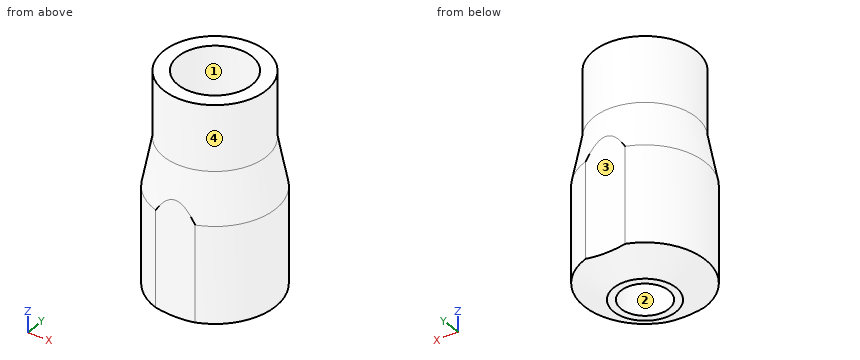
from build123d import *

# Parameters (mm, degrees)
SKETCH1_R           = 5.2451
BOSS_EXTRUDE1_DEPTH = 9.7155
CHAMFER1_SIZE       = 2.54
CHAMFER1_SIZE2      = 1.407944991
SKETCH2_R           = 4.445
SKETCH3_R           = 4.445
BOSS_EXTRUDE2_DEPTH = 5.6515
SKETCH4_R           = 2.069853247
CUT_EXTRUDE1_DEPTH  = 13.7795
SKETCH5_OUTSIDE_W   = 17.394
SKETCH5_OUTSIDE_H   = 17.394
SKETCH5_OUTSIDE_W_2 = 15.169695532
SKETCH5_OUTSIDE_H_2 = 9.924235678
CUT_EXTRUDE2_DEPTH  = 11.7475
SKETCH6_R           = 3.20242673
CUT_EXTRUDE3_DEPTH  = 8.1915


with BuildPart() as part:
    # Sketch1 → Boss-Extrude1 (new body)
    with BuildSketch(Plane.XY):
        with Locations(Location((0, 0, 0), (0, 0, 180))):
            Circle(SKETCH1_R)
    extrude(amount=BOSS_EXTRUDE1_DEPTH)

    # Chamfer1
    chamfer1_edges = [part.edges().sort_by_distance(p)[0] for p in [
        (5.2451, 0, 0),
    ]]
    chamfer1_side = [part.faces().sort_by_distance(p)[0] for p in [
        (0, 0, 0),
    ]]
    chamfer(chamfer1_edges, length=CHAMFER1_SIZE, length2=CHAMFER1_SIZE2, reference=chamfer1_side[0])

    # Sketch2 → section 1 of loft1
    with BuildSketch(Plane.XY.offset(13.8684), mode=Mode.PRIVATE) as loft1_s1:
        Circle(SKETCH2_R)
    # loft up to a face of the part (loft1)
    loft([Face(Wire([part.edges().sort_by_distance((3.590518025, -3.823513348, 9.7155))[0]])), loft1_s1.sketch])

    # Sketch3 → Boss-Extrude2 (add)
    with BuildSketch(Plane.XY.offset(13.8684)):
        with Locations(Location((0, 0, 0), (0, 0, 180))):
            Circle(SKETCH3_R)
    extrude(amount=BOSS_EXTRUDE2_DEPTH)

    # Sketch4 → Cut-Extrude1 (cut)
    with BuildSketch(Plane(origin=(0, 0, 0), x_dir=(-1, 0, 0), z_dir=(0, 0, -1))):
        Circle(SKETCH4_R)
    extrude(amount=-CUT_EXTRUDE1_DEPTH, mode=Mode.SUBTRACT)

    # Sketch5 outside → Cut-Extrude2 (cut)
    with BuildSketch(Plane.XY):
        Rectangle(SKETCH5_OUTSIDE_W, SKETCH5_OUTSIDE_H)
        with Locations((-0.203425036, 0)):
            Rectangle(SKETCH5_OUTSIDE_W_2, SKETCH5_OUTSIDE_H_2, mode=Mode.SUBTRACT)
    extrude(amount=CUT_EXTRUDE2_DEPTH, mode=Mode.SUBTRACT)

    # Sketch6 → Cut-Extrude3 (cut)
    with BuildSketch(Plane.XY.offset(19.5199)):
        Circle(SKETCH6_R)
    extrude(amount=-CUT_EXTRUDE3_DEPTH, mode=Mode.SUBTRACT)


solid = part.part
Can you work these out from the model? Positions are in its coordinate system, mm. Face numbers are marked on the shaded views. Give positions to 0.01 mm unless a question says otherwise; leave off trailing zeros. Order: outer loops, then holes, each group sorted by start corner. A loop starts at its lowest first (then second) coordinate and runs counter-clockwise, first axis right, second up. Notation, with made-up numbers: M 78,-22.75 L 127,-22.75 A9 cw 127,-9.75 Z; hole C 82,-15.5 d11. An arc over 180 degrees is marked long. Use a Markdown table: item, result. Add a question column.
Item 1: If I drill on L1, parallel to Y at x = 0, z = 2.5; L2, parallel to Y at x = 0, z = 16.5 (3 decimals); L3, parallel to Z at x = 2.5, y = -1, over which ranges is the centre line in solid material (lowest first)? Write a range as [from, to].
Item 2: Suppose I cut it at A-A (x = 0). List the corners of the cut face in (y, z) for me (3 decimals), then the cut area to 3 significant figures.
Item 3: Suppose I cut it at C-C (z = 18.25). List the corners of the cut face in (x, y) for me (3 decimals).
Item 4: Suppose I cut it at B-B (z = 9.5). List the corners of the cut face in (x, y) for me, then the cut area to 3 significant figures.
Item 5: We'd pull the mould along X, two halves only. Please class the marked faces 1, 2, 3 and 4: +X half, -X half, draft (parallel to the pull), parting line (faces both ways), or undercut.
Item 6: Will these pins go through, and if not, where does the flat tip stop? pin 1 (2 mm diameter, centred on y = 3.5, z = 2.5, fed in from +X); pin 2 (4 mm diameter, centred on y = -3.5, z = 10, fed in from -X); pin 3 (1 mm diameter, centred on y = 3.5, z = 14, fed in from -X).
Answer sheet:
| question | item | result |
|---|---|---|
| 1 | L1 | y = [-4.96, -2.07], [2.07, 4.96] |
| 1 | L2 | y = [-4.445, -3.202], [3.202, 4.445] |
| 1 | L3 | z = [0, 11.33] |
| 2 | outline | M -4.962,1.251 L -2.705,0 L -2.07,0 L -2.07,11.328 L -3.202,11.328 L -3.202,19.52 L -4.445,19.52 L -4.445,13.868 L -4.962,11.184 Z; M 2.07,0 L 2.705,0 L 4.962,1.251 L 4.962,11.184 L 4.445,13.868 L 4.445,19.52 L 3.202,19.52 L 3.202,11.328 L 2.07,11.328 Z |
| 2 | area | 84.3 mm² |
| 3 | outline | C 0,0 d8.89; hole C 0,0 d6.405 |
| 4 | outline | M -1.7,-4.96 L 1.7,-4.96 A5.25 ccw 1.7,4.96 L -1.7,4.96 A5.25 ccw Z; hole C 0,0 d4.14 |
| 4 | area | 71.7 mm² |
| 5 | face 1 | undercut |
| 5 | face 2 | undercut |
| 5 | face 3 | draft |
| 5 | face 4 | parting line |
| 6 | pin 1 | stops at x = 4.61 |
| 6 | pin 2 | stops at x = -5.02 |
| 6 | pin 3 | stops at x = -3.28 |
